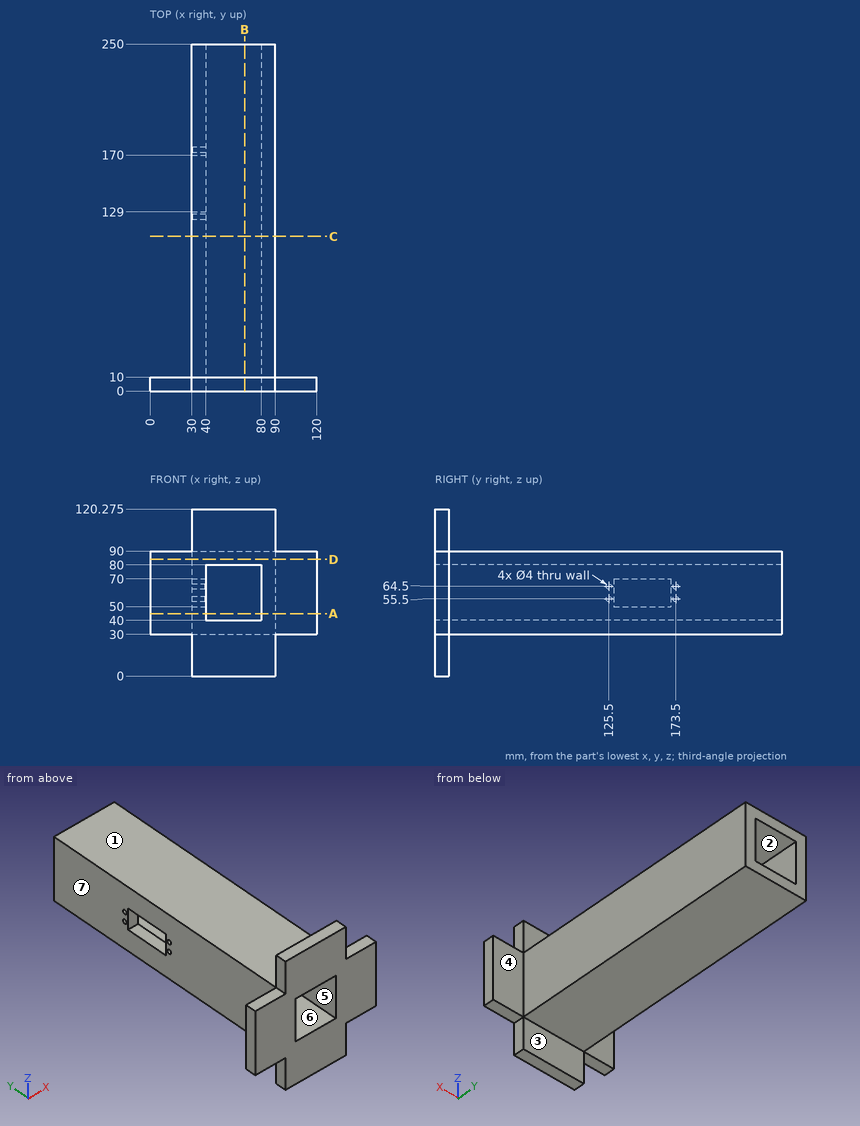
Geometry: see drawing. Coordinates: mm, zero at the bounding-box minimum. A direction names the side the tool comes from. Give positions to 0.01 mm unless a question says otherwise; leave off trailing zeros. Order: outer loops, then holes, each group sorted by start corner. A loop starts at its lowest first (then second) coordinate and runs counter-clockwise, first axis right, second up. Notation, with made-up numbers: (-37, -28) - (6, -28) arc R11 cw to (6, -13) - close; hole circle Ø2 at (63.25, -29.75). An arc over 180 degrees is marked (long way). Use CSV: the item, a comma, the result in double quotes.
1. Access query for the marked faces 1, 2 and 3. Directions: +Z, -Z, +X, -X, +Y, -Y. A direction counts if a zero-diameter tool reaches every point of the face in a straight line with its end or side. Return the directions, or none.
Answers below:
face 1,"+Z, +X, -X, +Y"
face 2,"+Y, -Y"
face 3,"-Z, +X, -X, +Y"
2. Section query B-B (x = 68). Output: boundary loops of the cut face in (y, z) (3 decimals).
Answers below:
outline,"(0, 0) - (10, 0) - (10, 30) - (250, 30) - (250, 40) - (0, 40) - close; (0, 80) - (250, 80) - (250, 90) - (10, 90) - (10, 120.275) - (0, 120.275) - close"
3. Contact query for flat-ended pins moving along their axis: pin 1 (3 mm diameter, centred on x = 35.5, z = 61, fed in from -Y); pin 2 (2 mm diameter, centred on y = 225, z = 32.5, fed in from +X); pin 3 (9 mm diameter, centred on x = 73, z = 8, fed in from +Y); pin 4 (10 mm diameter, centred on x = 23.5, z = 15, fed in from -Y). Output: stop coordinate, or through.
Answers below:
pin 1,"y = 0"
pin 2,"x = 90"
pin 3,"y = 10"
pin 4,"through"
4. Mould query, pull axis X, two halves, no side actions, for the marked faces 4, 5, 6 and 7. Classes: +X half, -X half, draft (parallel to the pull), parting line (faces both ways), or undercut.
Answers below:
face 4,"draft"
face 5,"undercut"
face 6,"undercut"
face 7,"-X half"
5. Section query D-D (z = 84). Output: boundary loops of the cut face in (x, y).
Answers below:
outline,"(0, 0) - (120, 0) - (120, 10) - (90, 10) - (90, 250) - (30, 250) - (30, 10) - (0, 10) - close"
6. Section query A-A (z = 45). Output: boundary loops of the cut face in (x, y), plus the area to 3 significant figures.
Answers below:
outline,"(0, 0) - (40, 0) - (40, 250) - (30, 250) - (30, 10) - (0, 10) - close; (80, 0) - (120, 0) - (120, 10) - (90, 10) - (90, 250) - (80, 250) - close"
area,"5,600 mm2"
7. Section query C-C (y = 111.5). Output: boundary loops of the cut face in (x, z), plus the area to 3 significant figures.
Answers below:
outline,"(30, 30) - (90, 30) - (90, 90) - (30, 90) - close; hole (40, 40) - (80, 40) - (80, 80) - (40, 80) - close"
area,"2,000 mm2"
8. Material intervals for line 1 along Y through (x, z) = (33.25, 64.5); line 2 along Z through (x, y) = (36.75, 173.5); line 3 along X through (y, z) = (201.5, 52), sorted ascending. Write a range as from..to.
Answers below:
line 1,"0..123.5, 127.5..129, 170..171.5, 175.5..250"
line 2,"30..53.5, 57.5..62.5, 66.5..90"
line 3,"30..40, 80..90"
